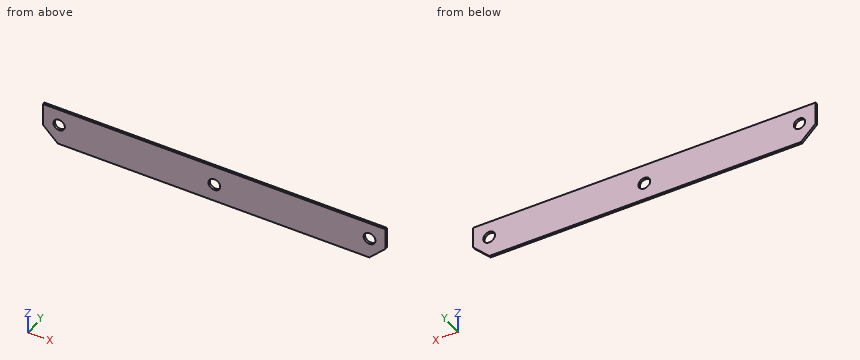
from build123d import *

# Parameters (mm, degrees)
SKETCH1_R           = 3.824987574
SKETCH1_R_2         = 3.960069723
SKETCH1_R_3         = 3.979490197
BOSS_EXTRUDE1_DEPTH = 1.5875


with BuildPart() as part:
    # Sketch1 → Boss-Extrude1 (new body)
    with BuildSketch(Plane(origin=(0, 0, 0), x_dir=(1, 0, 0), z_dir=(0, 1, 0))):
        Polygon((9.878524394, 25.4), (0, 15.521475606), (0, 0), (230, 0), (230, 14.509954572), (219.109954572, 25.4), align=None)
        with Locations(Location((10.82729629, 11.29561028, 0), (0, 0, 270))):
            Circle(SKETCH1_R, mode=Mode.SUBTRACT)
        with Locations(Location((219.17270371, 11.29561028, 0), (0, 0, 270))):
            Circle(SKETCH1_R_2, mode=Mode.SUBTRACT)
        with Locations(Location((115, 13.4, 0), (0, 0, 270))):
            Circle(SKETCH1_R_3, mode=Mode.SUBTRACT)
    extrude(amount=BOSS_EXTRUDE1_DEPTH)


solid = part.part
Here's how the part is built. I have some questions about the finished solid (model axes, mm). Coordinates: 2 decimals unless noted, no trailing zeros. Order: outer loops, then holes, each group sorted by start corner. A loop starts at its lowest first (then second) coordinate and runs counter-clockwise, first axis right, second up. Notation, with made-up numbers: (-12, -16.75) -> (47, -16.75) arc R18 cw to (47, 17.25) -> close; hole circle Ø2 at (9.25, 13.5). An arc over 180 degrees is marked (long way). Answer in a Markdown table with one row per item.
(1) I want a section at C-C on z = -21.5. List the corners of the cut face in (x, y) for me.
Answer key:
| item | result |
|---|---|
| outline | (5.98, 0) -> (223.01, 0) -> (223.01, 1.59) -> (5.98, 1.59) -> close |
(2) I want a section at B-B on y = 0.3. List the corners of the cut face in (x, z) for me.
Answer key:
| item | result |
|---|---|
| outline | (0, -15.52) -> (9.88, -25.4) -> (219.11, -25.4) -> (230, -14.51) -> (230, 0) -> (0, 0) -> close; hole circle Ø7.65 at (10.83, -11.3); hole circle Ø7.96 at (115, -13.4); hole circle Ø7.92 at (219.17, -11.3) |
(3) I want a section at A-A on x = 115. List the corners of the cut face in (y, z) for me.
Answer key:
| item | result |
|---|---|
| outline | (0, -25.4) -> (1.59, -25.4) -> (1.59, -17.38) -> (0, -17.38) -> close; (0, -9.42) -> (1.59, -9.42) -> (1.59, 0) -> (0, 0) -> close |
(4) Please list where these lines run through material, in increasing order: probe 1 along X at (y, z) = (0.8, -13.25); probe 2 along X at (y, z) = (0.9, -13.4); probe 3 along X at (y, z) = (1.3, -9.25).
Answer key:
| item | result |
|---|---|
| probe 1 | 0 to 7.54, 14.12 to 111.02, 118.98 to 215.73, 222.62 to 230 |
| probe 2 | 0 to 7.63, 14.02 to 111.02, 118.98 to 215.82, 222.53 to 230 |
| probe 3 | 0 to 7.6, 14.06 to 215.78, 222.56 to 230 |
(5) Will this pin go through, and if not, where does the flat tip stop? pin 1 Ø9 at (x, z) = (10.83, -11.3) entering from -Y.
Answer key:
| item | result |
|---|---|
| pin 1 | y = 0 |
